Check sheet for the drawn part. Datum: minimum x, y, z corner. Units: mm. Give positions to 0.01 mm unless a question says otherwise; leave off trailing zeros. Loops run counter-clockwise (first coordinate to the right, second up) from the corner with the lowest first, then second, coordinate; pieces in that order, holes last. Notation, with made-up numbers: M 87,55.25 L 113,55.25 A27 cw 113,89.25 Z; hole C 11,35.5 d2. An arc over 180 degrees is marked long. Write each question's results on one line, items separated by ' | '. Start each with the question number.
1. Sectioned sample at C-C on y = 58. Record the cut outline in (x, z), and give its area (3 significant figures).
2. Sectioned sample at D-D on y = 5. Record the cut outline in (x, z), and give its area (3 significant figures).
3. Sectioned sample at B-B on z = 7.5. Record the cut outline in (x, y).
4. Draft check along Y on the marked faces 1, 2, 3 and 4. Enter one of: pulls with the +Y half, pulls with the -Y half, needs draft (parallel to the pull), parting line crosses it, or undercut.
5. Material ranges on line 1 along X through (y, z) = (25, 1.6); line 2 along X through (y, z) = (44.5, 4.5); line 3 along Z through (x, y) = (25, 84), recorded low to high.
6. Sectioned sample at A-A on y = 45. Record the cut outline in (x, z), and give its area (3 significant figures).
7. Go/stop test with flat-tipped pins: pin 1 (6 mm diameter, centred on x = 52, z = 7.5, fed in from -Y); pin 2 (4 mm diameter, centred on x = 24.5, y = 25, fed in from -Z); pin 3 (8 mm diameter, centred on x = 33, z = 8, fed in from +Y). Record where each tip stops, or that it passes through.
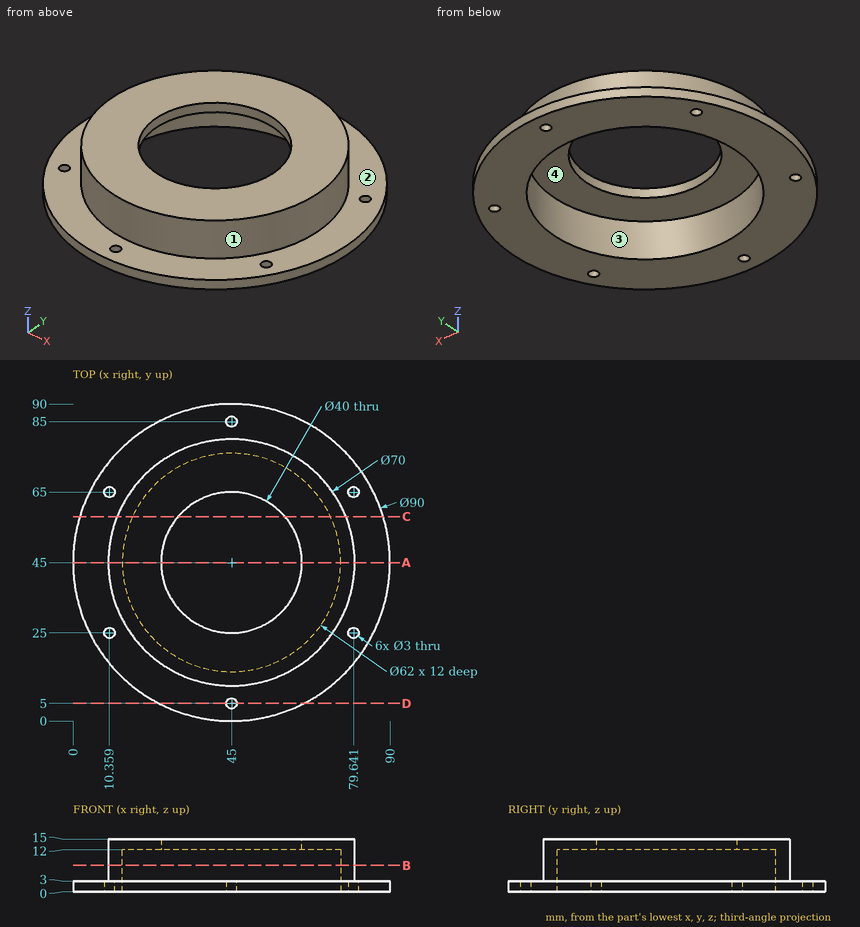
Output values:
1) outline: M 1.92,0 L 16.86,0 L 16.86,12 L 29.8,12 L 29.8,15 L 12.5,15 L 12.5,3 L 1.92,3 Z; M 60.2,12 L 73.14,12 L 73.14,0 L 88.08,0 L 88.08,3 L 77.5,3 L 77.5,15 L 60.2,15 Z | area: 272 mm2
2) outline: M 24.38,0 L 43.5,0 L 43.5,3 L 24.38,3 Z; M 46.5,0 L 65.62,0 L 65.62,3 L 46.5,3 Z | area: 115 mm2
3) outline: C 45,45 d70; hole C 45,45 d62
4) face 1: parting line crosses it | face 2: needs draft | face 3: undercut | face 4: undercut
5) line 1: 4.69 to 8.86, 11.86 to 21.31, 68.69 to 78.14, 81.14 to 85.31 | line 2: 10 to 14, 76 to 80 | line 3: 0 to 3
6) outline: M 0,0 L 14,0 L 14,12 L 25,12 L 25,15 L 10,15 L 10,3 L 0,3 Z; M 65,12 L 76,12 L 76,0 L 90,0 L 90,3 L 80,3 L 80,15 L 65,15 Z | area: 246 mm2
7) pin 1: y = 10.23 | pin 2: z = 12 | pin 3: y = 79.07
